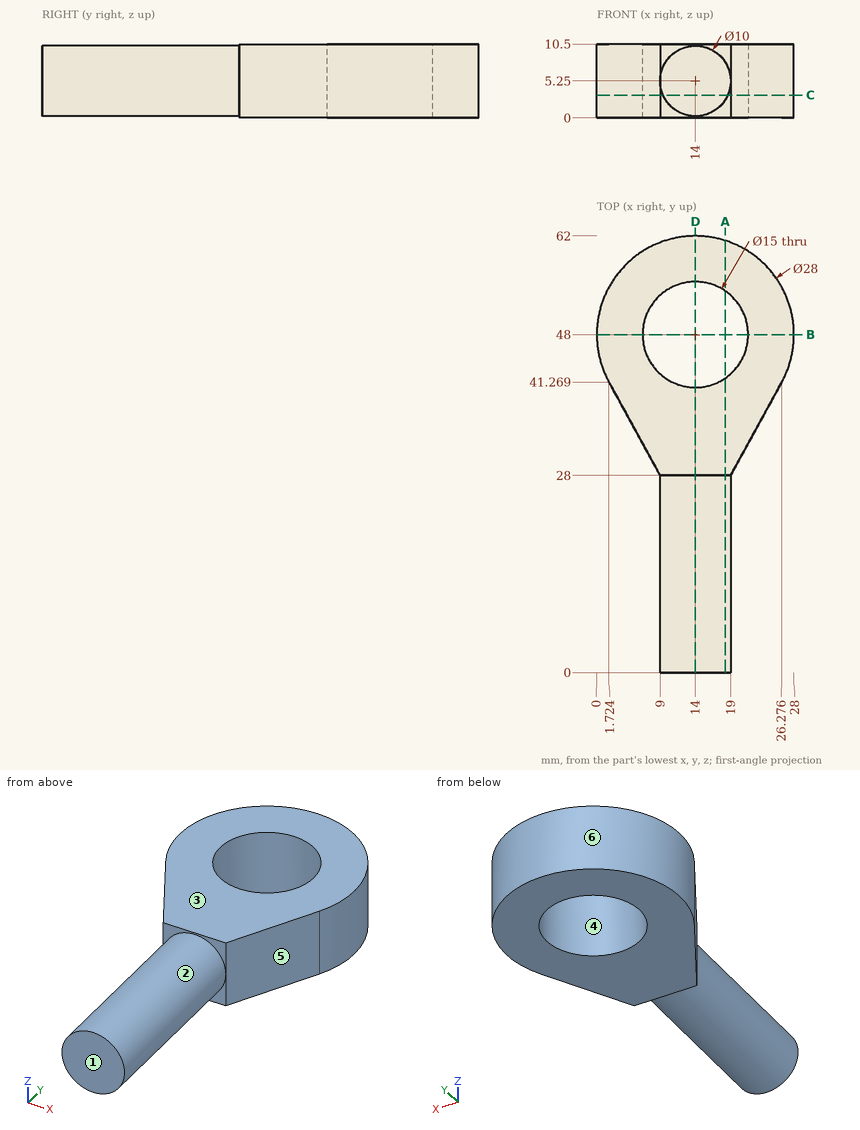
Check sheet for the drawn part. Datum: minimum x, y, z corner. Units: mm. A direction names the side the tool comes from. Give positions to 0.01 mm unless a question says otherwise; leave off trailing zeros. Order: outer loops, then holes, each group sorted by start corner. A loop starts at its lowest first (then second) coordinate and runs counter-clockwise, first axis right, second up.
1. Sectioned sample at B-B (y = 48). Record the boundary of the cut face in (x, z), then the cut area to 4 significant figures.
Completed:
outline: (0, 0) - (6.5, 0) - (6.5, 10.5) - (0, 10.5) - close; (21.5, 0) - (28, 0) - (28, 10.5) - (21.5, 10.5) - close
area: 136.5 mm2
2. Access from +Z, -Z, +X, -X, +Y, -Y to the whole of each face (thin tool, end or side, straight path). Record for the marked faces 1 and 2.
Completed:
face 1: +Z, -Z, +X, -X, -Y
face 2: -Y
3. Sectioned sample at D-D (x = 14). Record the boundary of the cut face in (y, z).
Completed:
outline: (0, 0.25) - (28, 0.25) - (28, 0) - (40.5, 0) - (40.5, 10.5) - (28, 10.5) - (28, 10.25) - (0, 10.25) - close; (55.5, 0) - (62, 0) - (62, 10.5) - (55.5, 10.5) - close
4. Sectioned sample at A-A (x = 18.25). Record the boundary of the cut face in (y, z), then the cut area to 3 significant figures.
Completed:
outline: (0, 2.62) - (28, 2.62) - (28, 0) - (41.82, 0) - (41.82, 10.5) - (28, 10.5) - (28, 7.88) - (0, 7.88) - close; (54.18, 0) - (61.34, 0) - (61.34, 10.5) - (54.18, 10.5) - close
area: 368 mm2
5. Scan lines: line 1 (Y direction, x = 14, z = 7.5); line 2 (X direction, y = 53.5, z = 5) (1 decimal); line 3 (Y direction, x = 10.5, z = 1.75) (1 decimal). Record each from-to range of solid material in increasing order.
Completed:
line 1: y = 0 to 40.5, 55.5 to 62
line 2: x = 1.1 to 8.9, 19.1 to 26.9
line 3: y = 0 to 41.4, 54.6 to 61.6
6. Depth check by flat-ended pin: pin 1 (2 mm diameter, centred on x = 7, z = 1.5, fed in from -Y) (1 decimal); pin 2 (6 mm diameter, centred on y = 19.5, z = 2, fed in from +X); pin 3 (6 mm diameter, centred on y = 54.5, z = 5, fed in from +X) (1 decimal). Enter the tip coordinate at first touch or a pass-through.
Completed:
pin 1: stops at y = 29.8
pin 2: stops at x = 18.99
pin 3: stops at x = 27.6
7. Draft check along Y on the marked faces 3, 4, 5 and 6. Enter one of: pulls with the +Y half, pulls with the -Y half, needs draft (parallel to the pull), parting line crosses it, or undercut.
Completed:
face 3: needs draft
face 4: undercut
face 5: pulls with the -Y half
face 6: parting line crosses it
8. Sectioned sample at C-C (z = 3.25). Record the boundary of the cut face in (x, y).
Completed:
outline: (1.72, 41.27) - (9, 28) - (9.42, 28) - (9.42, 0) - (18.58, 0) - (18.58, 28) - (19, 28) - (26.28, 41.27) arc R14 ccw (long way) to start; hole circle Ø15 at (14, 48)
